Design review of the part built by this model. Coordinates are the model's own, in mm. A direction names the side the tool comes from. Coordinates: 2 decimals unless noted, no trailing zeros. Loops run counter-clockwise (first coordinate to the right, second up) from the corner with the lowest first, then second, coordinate; pieces in that order, holes last. Notation, with made-up numbers: (-17, -15.75) -> (39, -15.75) arc R7 cw to (39, -3.75) -> close; hole circle Ø10 at (69, 37.25). An arc over 180 degrees is marked (long way). Use one line per item in the form item = value. Start each with the question number.
1. Consider section B-B (x = 0). State the section outline as (y, z) points (3 decimals), then the cut area to 3 significant figures.
2. Consider section D-D (z = -7). State the section outline as (x, y) points (3 decimals).
3. For pin 1 (3 mm diameter, centred on x = 0, z = 0, fed in from -Y); pin 2 (6.5 mm diameter, centred on x = -0.5, z = 3, fed in from -Y), all flat-tipped, find the tip position at first contact; note any pin that passes through.
4. Machinability: for faces 1 (the face through (3.38, -0.61, 3.21)), 2 (the face through (0, 0, 0)), 3 (the face through (0, -2, 7.925)), which of the approach directions +Z, -Z, +X, -X, +Y, -Y give a long, thin tool a straight path to every point of the face, cutting with its end or side? Answer none if there is none.
5. Wall thickness on line 1 (X direction, y = -2.5, z = 0) (3 decimals); line 2 (Z direction, x = -3.75, y = -0.3) (3 decimals); line 3 (Z direction, x = 4.25, y = -0.45) (3 decimals): over which ranges is each line inside the solid? List them lowest first. Write a range as from..to.
6. Consider section C-C (y = 0.65). State the section outline as (x, z) points.
7. The part is to be moulded in two halves that separate along X. For faces 4 (the face through (0, -1.5, 0)), 5 (the face through (-4, 1.8, -4)), 6 (the face through (4, 0.3, -4)), say which applies: released by +X, released by -X, zero draft, split by the parting line, or undercut.
8. Consider section A-A (z = 0). State the section outline as (x, y) points (3 decimals).
from build123d import *

# Parameters (mm, degrees)
SKETCH1_W           = 15.85
SKETCH1_H           = 15.85
BOSS_EXTRUDE1_DEPTH = 3.15
SKETCH2_R           = 2.45
BOSS_EXTRUDE2_DEPTH = 1.8
SHELL1_T            = -1.5
SKETCH3_R           = 3.25
SKETCH3_R_2         = 2.45
BOSS_EXTRUDE3_DEPTH = 1.45


with BuildPart() as part:
    # Sketch1 → Boss-Extrude1 (new body)
    with BuildSketch(Plane(origin=(0, 0, 0), x_dir=(1, 0, 0), z_dir=(0, 1, 0))):
        Rectangle(SKETCH1_W, SKETCH1_H)
    extrude(amount=-BOSS_EXTRUDE1_DEPTH)

    # Sketch2 → Boss-Extrude2 (add)
    with BuildSketch(Plane(origin=(0, 0, 0), x_dir=(1, 0, 0), z_dir=(0, 1, 0))):
        with Locations(Location((-3.9625, 3.9625, 0), (0, 0, 270))):
            Circle(SKETCH2_R)
        with Locations(Location((-3.9625, -3.9625, 0), (0, 0, 270))):
            Circle(SKETCH2_R)
        with Locations(Location((3.9625, 3.9625, 0), (0, 0, 270))):
            Circle(SKETCH2_R)
        with Locations(Location((3.9625, -3.9625, 0), (0, 0, 270))):
            Circle(SKETCH2_R)
    extrude(amount=BOSS_EXTRUDE2_DEPTH)

    # Shell1
    shell1_openings = [part.faces().sort_by_distance(p)[0] for p in [
        (0, -3.15, 0),
    ]]
    offset(amount=SHELL1_T, openings=shell1_openings, kind=Kind.INTERSECTION)

    # Sketch3 → Boss-Extrude3 (add)
    with BuildSketch(Plane.XZ.offset(1.5)):
        with Locations(Location((0, 0, 0), (0, 0, 90))):
            Circle(SKETCH3_R)
        with Locations(Location((0, 0, 0), (0, 0, 90))):
            Circle(SKETCH3_R_2, mode=Mode.SUBTRACT)
    extrude(amount=BOSS_EXTRUDE3_DEPTH)


solid = part.part
Geometry check:
q1.outline = (-3.15, -7.925) -> (0, -7.925) -> (0, 7.925) -> (-3.15, 7.925) -> (-3.15, 6.425) -> (-1.5, 6.425) -> (-1.5, 3.25) -> (-2.95, 3.25) -> (-2.95, 2.45) -> (-1.5, 2.45) -> (-1.5, -2.45) -> (-2.95, -2.45) -> (-2.95, -3.25) -> (-1.5, -3.25) -> (-1.5, -6.425) -> (-3.15, -6.425) -> close
q1.area = 31.0 mm²
q2.outline = (-7.925, -3.15) -> (7.925, -3.15) -> (7.925, 0) -> (-7.925, 0) -> close
q3.pin_1 = -1.5
q3.pin_2 = -2.95
q4.face_1 = -Y
q4.face_2 = +Y
q4.face_3 = +Z, +X, -X, +Y, -Y
q5.line_1 = -7.925..-6.425, -3.25..-2.45, 2.45..3.25, 6.425..7.925
q5.line_2 = -7.925..-4.888, -3.037..3.037, 4.888..7.925
q5.line_3 = -7.925..-4.868, -3.057..3.057, 4.868..7.925
q6.outline = circle Ø4.9 at (-3.96, -3.96); circle Ø4.9 at (-3.96, 3.96); circle Ø4.9 at (3.96, -3.96); circle Ø4.9 at (3.96, 3.96)
q7.face_4 = undercut
q7.face_5 = zero draft
q7.face_6 = undercut
q8.outline = (-7.925, -3.15) -> (-6.425, -3.15) -> (-6.425, -1.5) -> (-3.25, -1.5) -> (-3.25, -2.95) -> (-2.45, -2.95) -> (-2.45, -1.5) -> (2.45, -1.5) -> (2.45, -2.95) -> (3.25, -2.95) -> (3.25, -1.5) -> (6.425, -1.5) -> (6.425, -3.15) -> (7.925, -3.15) -> (7.925, 0) -> (-7.925, 0) -> close
